Can you work these out from the model? Positions are in its coordinate system, mm. Coordinates: 2 decimals unless noted, no trailing zeros. Order: outer loops, then holes, each group sorted by start corner. A loop starts at its lowest first (then second) coordinate and runs counter-clockwise, first axis right, second up. Notation, with made-up numbers: (7, 40) -> (55, 40) arc R18 ccw to (55, 44) -> close; hole circle Ø1 at (59.5, -10.75). An arc over 180 degrees is marked (long way). Answer in a Markdown table with one row per item. Add a question column.
1. Imagine slicing it at B-B on z = 5.5. Write out the boundary of the cut face in (x, y), plus the area to 3 significant figures.
2. Imagine slicing it at A-A on y = 0. Write out the boundary of the cut face in (x, z) (3 decimals), plus the area to 3 significant figures.
3. If I drill on line 1 along Y through (x, z) = (-1.5, -6.5); line 2 along Y through (x, z) = (1.35, -4); line 3 along X through (y, z) = (1.3, -3.75), over which ranges is the centre line in solid material (lowest first)? Write a range as [from, to].
4. Imagine slicing it at C-C on y = -1. State how many separate pieces and enclosed holes the cut face has, plus the area to 3 significant figures.
5. We'd pull the mould along Y, two halves only. Please class faces 1 (the face through (-0.781, -0.304, 0.133)), 2 (the face through (-1.63, -0.25, 0.12)), 3 (the face through (0, 1, -9.525)): pulls with the +Y half, pulls with the -Y half, needs draft (parallel to the pull), parting line crosses it, or undercut.
from build123d import *

# Parameters (mm, degrees)
EXTRUDE_THIN1_DEPTH = 9.525


with BuildPart() as part:
    # Sketch2 → Extrude-Thin1 (new, symmetric)
    with BuildSketch(Plane.XY):
        with BuildLine():
            ThreePointArc((0, 1.651), (-1.6259176, -0.286693141), (0.564675257, -1.551432517))
            ThreePointArc((0.564675257, -1.551432517), (1.428087859, 0.300161785), (-0.423506442, 1.163574388))
            ThreePointArc((-0.423506442, 1.163574388), (-1.163574388, -0.423506442), (0.423506442, -1.163574388))
            ThreePointArc((0.423506442, -1.163574388), (1.010514268, 0.218497398), (-0.408926516, 0.708281502))
            Line((-0.408926516, 0.708281502), (-0.22127156, 0.354615342))
            ThreePointArc((-0.22127156, 0.354615342), (0.644689881, 0.055811649), (0.286572693, -0.787352002))
            ThreePointArc((0.286572693, -0.787352002), (-0.787352002, -0.286572693), (-0.286572693, 0.787352002))
            ThreePointArc((-0.286572693, 0.787352002), (1.051865474, 0.163228035), (0.427741507, -1.175210132))
            ThreePointArc((0.427741507, -1.175210132), (-1.231632582, -0.217170055), (0, 1.2506325))
            Line((0, 1.2506325), (0, 1.651))
        make_face()
    extrude(amount=EXTRUDE_THIN1_DEPTH, both=True)

    # Sketch3 → Cut-Revolve1 (revolve, cut)
    with BuildSketch(Plane(origin=(0, 0, 0), x_dir=(0, 0, -1), z_dir=(1, 0, 0))):
        Polygon((-9.525, 1.651), (-9.525, 1.5367), (-8.4074, 1.651), align=None)
        Polygon((8.4074, 1.651), (9.525, 1.651), (9.525, 1.5367), align=None)
    revolve(axis=Axis((0, 0, 0), (0, 0, 1)), mode=Mode.SUBTRACT)


solid = part.part
Answers follow:
| question | item | result |
|---|---|---|
| 1 | outline | (-0.42, 1.16) arc R1.24 ccw to (0.42, -1.16) arc R1.03 ccw (long way) to (-0.41, 0.71) -> (-0.22, 0.35) arc R0.63 cw (long way) to (0.29, -0.79) arc R0.84 cw to (-0.29, 0.79) arc R1.04 cw to (0.43, -1.18) arc R1.25 cw (long way) to (0, 1.25) -> (0, 1.65) arc R1.65 ccw (long way) to (0.56, -1.55) arc R1.44 ccw to start |
| 1 | area | 5.98 mm² |
| 2 | outline | (-1.651, -8.407) -> (-1.537, -9.525) -> (-1.251, -9.525) -> (-1.251, 9.525) -> (-1.537, 9.525) -> (-1.651, 8.407) -> close; (-1.238, -9.525) -> (-0.838, -9.525) -> (-0.838, 9.525) -> (-1.238, 9.525) -> close; (0.666, -9.525) -> (1.08, -9.525) -> (1.08, 9.525) -> (0.666, 9.525) -> close; (1.097, -9.525) -> (1.502, -9.525) -> (1.502, 9.525) -> (1.097, 9.525) -> close |
| 2 | area | 30.7 mm² |
| 3 | line 1 | y = [-0.69, 0.69] |
| 3 | line 2 | y = [-0.86, 0.48] |
| 3 | line 3 | x = [-1.02, 0] |
| 4 | separate pieces | 3 |
| 4 | enclosed holes | 0 |
| 4 | area | 48.2 mm² |
| 5 | face 1 | undercut |
| 5 | face 2 | parting line crosses it |
| 5 | face 3 | needs draft |
